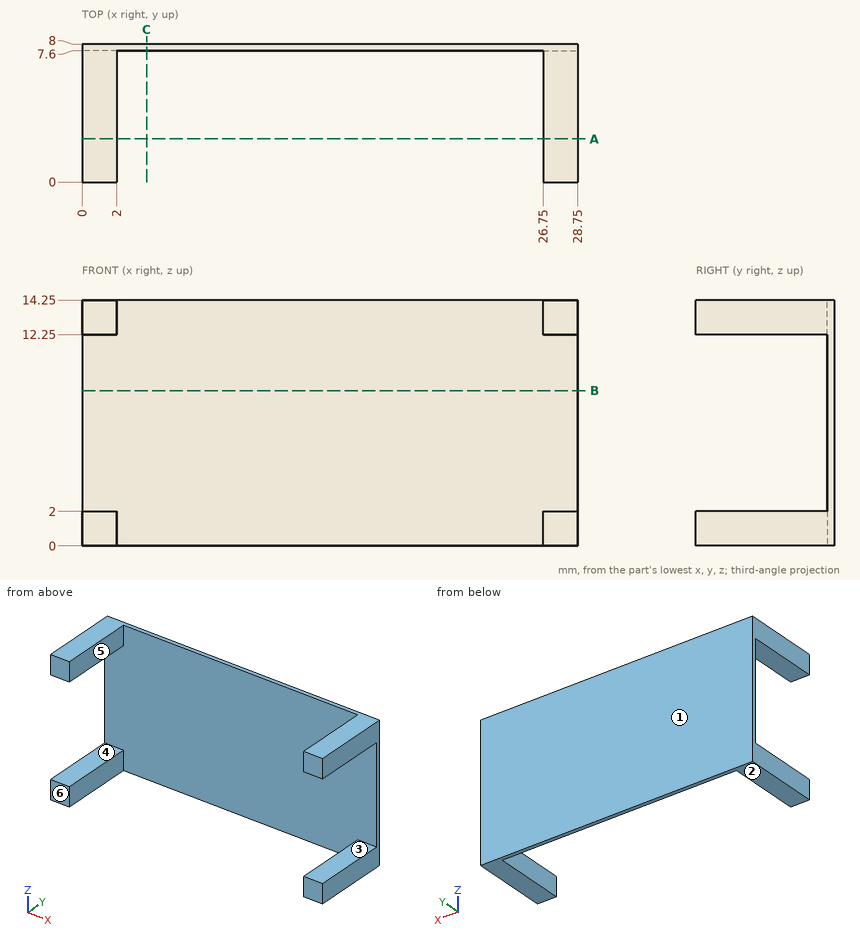
Check sheet for the drawn part. Datum: minimum x, y, z corner. Units: mm. A direction names the side the tool comes from. Give positions to 0.01 mm unless a question says otherwise; leave off trailing zeros. Loops run counter-clockwise (first coordinate to the right, second up) from the corner with the lowest first, then second, coordinate; pieces in that order, holes last.
1) Depth check by flat-ended pin: pin 1 Ø5 at (x, z) = (19.5, 5) entering from -Y. Enter the tip coordinate at first touch or a pass-through.
2) Sectioned sample at C-C, the plane x = 3.75. Enter the section's corners in (y, z), then the cut area to 3 significant figures.
3) Sectioned sample at A-A, the plane y = 2.5. Enter the section's corners in (x, z), then the cut area to 3 significant figures.
4) Sectioned sample at B-B, the plane z = 9. Enter the section's corners in (x, y), then the cut area to 3 significant figures.
5) Thickness scan on line 1 along X through (y, z) = (4.5, 1.75); line 2 along Z through (x, y) = (27.5, 3.25); line 3 along Y through (x, z) = (23, 9.75). Record the ranges inside material, lowest first.
6) Set-up check for the marked faces 4, 5 and 6: record each of +Z, -Z, +X, -X, +Y, -Y from which the full face is reachable in a straight line by a thin tool's end or side.
7) Draft check along Z on the marked faces 1, 2 and 3. Enter one of: pulls with the +Z half, pulls with the -Z half, needs draft (parallel to the pull), parting line crosses it, or undercut.
Answers:
1. pin 1: stops at y = 7.6
2. outline: (7.6, 0) - (8, 0) - (8, 14.25) - (7.6, 14.25) - close
2. area: 5.70 mm2
3. outline: (0, 0) - (2, 0) - (2, 2) - (0, 2) - close; (0, 12.25) - (2, 12.25) - (2, 14.25) - (0, 14.25) - close; (26.75, 0) - (28.75, 0) - (28.75, 2) - (26.75, 2) - close; (26.75, 12.25) - (28.75, 12.25) - (28.75, 14.25) - (26.75, 14.25) - close
3. area: 16.0 mm2
4. outline: (0, 7.6) - (28.75, 7.6) - (28.75, 8) - (0, 8) - close
4. area: 11.5 mm2
5. line 1: x = 0 to 2, 26.75 to 28.75
5. line 2: z = 0 to 2, 12.25 to 14.25
5. line 3: y = 7.6 to 8
6. face 4: +X, -X, -Y
6. face 5: +Z, -Z, -Y
6. face 6: +Z, -Z, +X, -X, -Y
7. face 1: needs draft
7. face 2: pulls with the -Z half
7. face 3: undercut
